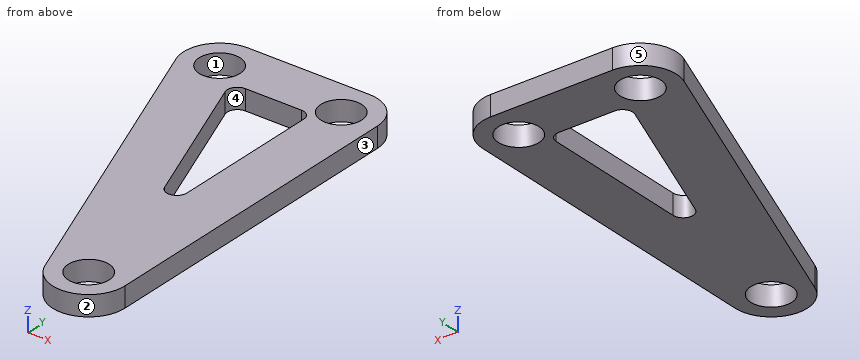
from build123d import *

# Parameters (mm, degrees)
ESQUISSE1_R        = 6.4135
BOSS_EXTRU_1_DEPTH = 6.35
CONG_1_R           = 3.175


with BuildPart() as part:
    # Esquisse1 → Boss.-Extru.1 (new body)
    with BuildSketch(Plane.XY):
        with BuildLine():
            Line((-10.583328694, -3.96874826), (27.516671306, -105.56874826))
            ThreePointArc((27.516671306, -105.56874826), (40.116735576, -112.721626977), (49.403, -101.6))
            Line((49.403, -101.6), (49.403, 0))
            ThreePointArc((49.403, 0), (46.092427948, 7.992427948), (38.1, 11.303))
            Line((38.1, 11.303), (0, 11.303))
            ThreePointArc((0, 11.303), (-9.290225255, 6.438130451), (-10.583328694, -3.96874826))
        make_face()
        Circle(ESQUISSE1_R, mode=Mode.SUBTRACT)
        with Locations((38.1, 0)):
            Circle(ESQUISSE1_R, mode=Mode.SUBTRACT)
        with Locations((38.1, -101.6)):
            Circle(ESQUISSE1_R, mode=Mode.SUBTRACT)
        Polygon((7.513703438, -5.207), (32.893, -72.885124166), (32.893, -5.207), align=None, mode=Mode.SUBTRACT)
    extrude(amount=BOSS_EXTRU_1_DEPTH)

    # Congé1
    cong_1_edges = [part.edges().sort_by_distance(p)[0] for p in [
        (32.893, -5.207, 3.175),
        (7.513703438, -5.207, 3.175),
        (32.893, -72.885124166, 3.175),
    ]]
    fillet(cong_1_edges, radius=CONG_1_R)


solid = part.part
Here's how the part is built. I have some questions about the finished solid (model axes, mm). Face numbers are marked on the shaded views. A direction names the side the tool comes from. Round coordinates to 2 decimals unless told otherwise and drop trailing zeros. Order: outer loops, then holes, each group sorted by start corner. A loop starts at its lowest first (then second) coordinate and runs counter-clockwise, first axis right, second up. Notation, with made-up numbers: M 42.25,56 L 60.25,56 A23 ccw 60.25,88 Z; hole C 44.5,47.25 d5. An arc over 180 degrees is marked long. Return JSON: item names as keys, results as strings. Group by question number.
1. On a 3-axis mill with a long thin cutter (end or side, diameter ignored), from which of +Z, -Z, +X, -X, +Y, -Y can I reach the whole of each face in a straight line? I mean the marked faces 4 and 5. Say none if no direction works.
2. I'm going to push flat-ended pins straight in: pin 1 Ø1 at (y, z) = (-57, 3.5) entering from -X; pin 2 Ø1.9 at (y, z) = (-23.5, 2.5) entering from -X. Where does each tip first touch, or does it pass through?
3. If we section it at A-A on y = -28: List the corners of the cut face in (x, z) for me, then the cut area to 3 significant figures.
4. If we section it at D-D on x = 15.5: List the corners of the cut face in (y, z) for me.
5. Please list where these lines run through material, in increasing order: probe 1 along Y at (x, z) = (38.1, 2); probe 2 along X at (y, z) = (0.5, 4.75); probe 3 along X at (y, z) = (-50.5, 0.75).
6. If we section it at C-C on x = 41.5: List the corners of the cut face in (y, z) for me.
7. If we mould it in two halves opening along Y, with no side actions, what happens to the marked faces 1, 2 and 3? For each: pulls with the +Y half, pulls with the -Y half, needs draft (parallel to the pull), parting line crosses it, or undercut.
8. If we section it at B-B on z = 2.5: State how many separate pieces and enclosed holes the cut face has, then the cut area to 3 significant figures.
Reply:
{
 "1": {"face 4": "+Z, -Z", "face 5": "+Z, -Z, -X"},
 "2": {"pin 1": "x = 9.12", "pin 2": "x = -3.62"},
 "3": {"outline": "M -1.57,0 L 16.06,0 L 16.06,6.35 L -1.57,6.35 Z; M 32.89,0 L 49.4,0 L 49.4,6.35 L 32.89,6.35 Z", "area": "217 mm^2"},
 "4": {"outline": "M -73.52,0 L -26.5,0 L -26.5,6.35 L -73.52,6.35 Z; M -5.21,0 L 11.3,0 L 11.3,6.35 L -5.21,6.35 Z"},
 "5": {"probe 1": "-112.9 to -108.01, -95.19 to -6.41, 6.41 to 11.3", "probe 2": "-11.29 to -6.39, 6.39 to 31.71, 44.49 to 49.39", "probe 3": "6.87 to 24.5, 32.89 to 49.4"},
 "6": {"outline": "M -112.38,0 L -107.04,0 L -107.04,6.35 L -112.38,6.35 Z; M -96.16,0 L -5.44,0 L -5.44,6.35 L -96.16,6.35 Z; M 5.44,0 L 10.78,0 L 10.78,6.35 L 5.44,6.35 Z"},
 "7": {"face 1": "undercut", "face 2": "pulls with the -Y half", "face 3": "needs draft"},
 "8": {"separate pieces": "1", "enclosed holes": "4", "area": "3,940 mm^2"}
}
